Source: three-view drawing plus pictorial views. Frame: mm from the lowest corner of the part. A direction names the side the tool comes from. Round coordinates to 2 decimals unless told otherwise and drop trailing zeros. Loops run counter-clockwise (first coordinate to the right, second up) from the corner with the lowest first, then second, coordinate; pieces in that order, holes last. Notation, with made-up numbers: (89.25, 16.25) -> (145.25, 16.25) arc R28 cw to (145.25, 43.25) -> close; hole circle Ø11 at (-9.5, 18.25). An arc over 180 degrees is marked (long way). Return JSON: item names as keys, results as strings. Group by question number.
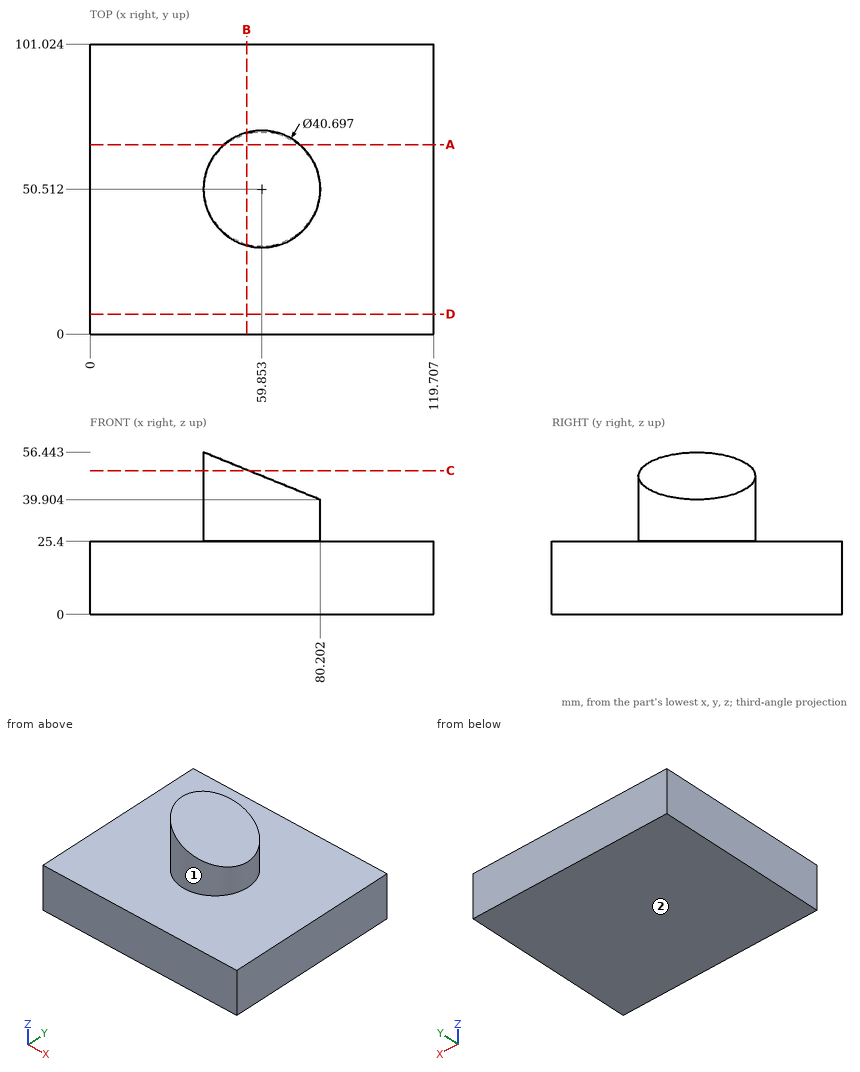
(1) Pin query (flat end, axial travel): pin 1 (6 mm diameter, centred on x = 107, y = 28.5, fed in from +Z); pin 2 (3 mm diameter, centred on x = 46, z = 43.5, fed in from +Y); pin 3 (12 mm diameter, centred on y = 50.5, z = 44.5, fed in from -X) (1 decimal). Return the tip coordinate at first contact, or that it passes through.
(2) Cut plane C-C (z = 50). Return loops of the section in (x, y), and give its area (3 significant figures).
(3) Cut plane A-A (y = 66). Return loops of the section in (x, z) (1 decimal), and give its area (3 significant figures).
(4) Cut plane D-D (y = 7). Return loops of the section in (x, z), and give its area (3 significant figures).
(5) Cut plane B-B (x = 54.5). Return loops of the section in (y, z), and give its area (3 significant figures).
(6) Set-up query: the marked faces 1 and 2. Return all of +Z, -Z, +X, -X, +Y, -Y with unobstructed straight access to the full face (end or side cutting, diameter ignored); none if empty.
(7) Ray query, line 1 (Z direction, x = 62, y = 18.5); line 2 (Y direction, x = 71, z = 39) (1 decimal); line 3 (X direction, y = 66.5, z = 34) (1 decimal). Return the intervals inside material, ascending.
Answers follow:
{
 "1": {"pin 1": "z = 25.4", "pin 2": "y = 66.68", "pin 3": "x = 39.5"},
 "2": {"outline": "(55.36, 30.67) -> (55.36, 70.36) arc R20.35 ccw to start", "area": "469 mm^2"},
 "3": {"outline": "(0, 0) -> (119.7, 0) -> (119.7, 25.4) -> (73.1, 25.4) -> (73.1, 42.8) -> (46.7, 53.5) -> (46.7, 25.4) -> (0, 25.4) -> close", "area": "3,640 mm^2"},
 "4": {"outline": "(0, 0) -> (119.71, 0) -> (119.71, 25.4) -> (0, 25.4) -> close", "area": "3,040 mm^2"},
 "5": {"outline": "(0, 0) -> (101.02, 0) -> (101.02, 25.4) -> (70.14, 25.4) -> (70.14, 50.35) -> (30.88, 50.35) -> (30.88, 25.4) -> (0, 25.4) -> close", "area": "3,550 mm^2"},
 "6": {"face 1": "+Z", "face 2": "-Z, +X, -X, +Y, -Y"},
 "7": {"line 1": "0 to 25.4", "line 2": "33.5 to 67.5", "line 3": "47.3 to 72.4"}
}
